Source: CAD feature listing. Evaluate the final solid. Frame: model axes, mm. A direction names the side the tool comes from. Coordinates: 2 decimals unless noted, no trailing zeros. Order: outer loops, then holes, each group sorted by start corner. A loop starts at its lowest first (then second) coordinate and runs counter-clockwise, first axis right, second up. Notation, with made-up numbers: (49.5, -1.75) -> (75.5, -1.75) arc R27 cw to (75.5, 29.25) -> close; hole circle Ø2 at (-13.5, 24.25). An arc over 180 degrees is marked (long way). Put each result on its own line as item: value.
from build123d import *

# Parameters (mm, degrees)
SKETCH2_W            = 35
SKETCH2_H            = 20.32
SKETCH2_R            = 4.572
BOSS_EXTRUDE1_DEPTH  = 48.26
M5_CLEARANCE_HOLE1_D = 5.5
SKETCH7_R            = 2.667
CUT_EXTRUDE1_DEPTH   = 5
SKETCH8_W            = 30
SKETCH8_H            = 25.4
CUT_EXTRUDE2_DEPTH   = 63.983569286


with BuildPart() as part:
    # Sketch2 → Boss-Extrude1 (new body)
    with BuildSketch(Plane(origin=(0, 0, 0), x_dir=(1, 0, 0), z_dir=(0, 1, 0))):
        with Locations((17.5, 10.16)):
            Rectangle(SKETCH2_W, SKETCH2_H)
        with Locations(Location((17.5, 10.16, 0), (0, 0, 90))):
            Circle(SKETCH2_R, mode=Mode.SUBTRACT)
    extrude(amount=BOSS_EXTRUDE1_DEPTH)

    # M5 Clearance Hole1 (through all)
    with Locations(Plane.XY):
        with Locations((5, 8.89), (30, 8.89)):
            Hole(M5_CLEARANCE_HOLE1_D / 2)

    # Sketch7 → Cut-Extrude1 (cut)
    with BuildSketch(Plane(origin=(0, 48.26, 0), x_dir=(1, 0, 0), z_dir=(0, 1, 0))):
        with Locations(Location((27.94, 3.81, 0), (0, 0, 270))):
            Circle(SKETCH7_R)
    extrude(amount=-CUT_EXTRUDE1_DEPTH, mode=Mode.SUBTRACT)

    # Sketch8 → Cut-Extrude2 (cut, through all)
    with BuildSketch(Plane(origin=(0, 0, -20.32), x_dir=(-1, 0, 0), z_dir=(0, 0, -1))):
        with Locations((-20, 27.94)):
            Rectangle(SKETCH8_W, SKETCH8_H)
    extrude(amount=-CUT_EXTRUDE2_DEPTH, mode=Mode.SUBTRACT)


solid = part.part
1. First-contact query: pin 1 (3 mm diameter, centred on y = 25.5, z = -2, fed in from -X); pin 2 (3 mm diameter, centred on x = 27.94, z = -3.81, fed in from +Y). Flat tips, straight axial feed; report the tip coordinate or a pass-through.
Numbers:
pin 1: stops at x = 0
pin 2: stops at y = 43.26
2. Pull-direction query (X, two-part tool) for faces 1 (the flat face through (13, 0, -13)), 2 (the flat face through (35, 44, -10)), 3 (the cylindrical face through (32.747, 9.011, -10.302)); classes: pulls with the +X half, pulls with the -X half, needs draft (parallel to the pull), parting line crosses it, or undercut.
Numbers:
face 1: needs draft
face 2: pulls with the +X half
face 3: undercut
3. Cut plane A-A on z = -10.16. Output: boundary loops of the cut face in (x, y), plus the area to 3 significant figures.
Numbers:
outline: (0, 0) -> (12.93, 0) -> (12.93, 15.24) -> (5, 15.24) -> (5, 40.64) -> (12.93, 40.64) -> (12.93, 48.26) -> (0, 48.26) -> close; (22.07, 0) -> (35, 0) -> (35, 15.24) -> (22.07, 15.24) -> close; (22.07, 40.64) -> (35, 40.64) -> (35, 48.26) -> (22.07, 48.26) -> close; hole circle Ø5.5 at (5, 8.89); hole circle Ø5.5 at (30, 8.89)
area: 671 mm2
4. Cut plane C-C on x = 10. Output: boundary loops of the cut face in (y, z), plus the area to 3 significant figures.
Numbers:
outline: (0, -20.32) -> (15.24, -20.32) -> (15.24, 0) -> (0, 0) -> close; (40.64, -20.32) -> (48.26, -20.32) -> (48.26, 0) -> (40.64, 0) -> close
area: 465 mm2
5. Cut plane D-D on x = 17.5. Output: boundary loops of the cut face in (y, z), plus the area to 3 significant figures.
Numbers:
outline: (0, -20.32) -> (15.24, -20.32) -> (15.24, -14.73) -> (0, -14.73) -> close; (0, -5.59) -> (15.24, -5.59) -> (15.24, 0) -> (0, 0) -> close; (40.64, -20.32) -> (48.26, -20.32) -> (48.26, -14.73) -> (40.64, -14.73) -> close; (40.64, -5.59) -> (48.26, -5.59) -> (48.26, 0) -> (40.64, 0) -> close
area: 255 mm2
6. Set-up query: faces 4 (the flat face through (24, 15.24, -10)), 5 (the flat face through (28, 43.26, -4)), 6 (the flat face through (0, 24, -10)). Return all of +Z, -Z, +X, -X, +Y, -Y with unobstructed straight access to the full face (end or side cutting, diameter ignored); none if empty.
Numbers:
face 4: +Z, -Z, +X
face 5: +Y
face 6: +Z, -Z, -X, +Y, -Y
7. Cut plane B-B on y = 8.89. Output: boundary loops of the cut face in (x, z), plus the area to 3 significant figures.
Numbers:
outline: (0, -20.32) -> (2.25, -20.32) -> (2.25, 0) -> (0, 0) -> close; (7.75, -20.32) -> (27.25, -20.32) -> (27.25, 0) -> (7.75, 0) -> close; (32.75, -20.32) -> (35, -20.32) -> (35, 0) -> (32.75, 0) -> close; hole circle Ø9.14 at (17.5, -10.16)
area: 422 mm2
8. Ray query, line 1 along Y through (x, z) = (22, -3.5); line 2 along Y through (x, z) = (30, -12.25); line 3 along X through (y, z) = (5, -10.16). Return the intervals inside material, ascending.
Numbers:
line 1: y = 0 to 15.24, 40.64 to 48.26
line 2: y = 0 to 6.14, 11.64 to 15.24, 40.64 to 48.26
line 3: x = 0 to 12.93, 22.07 to 35
